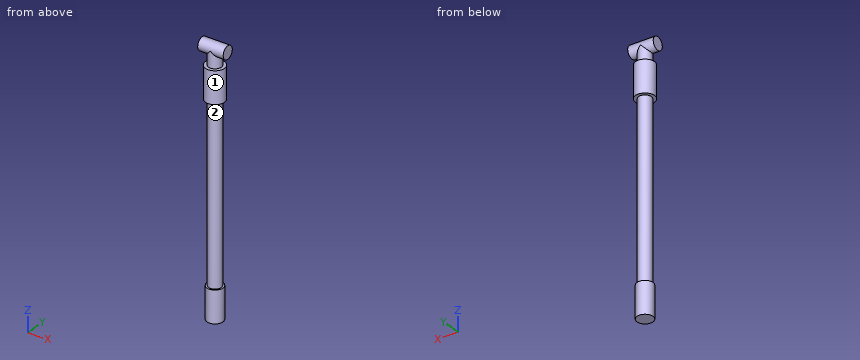
from build123d import *

# Parameters (mm, degrees)
SKETCH1_R                = 4
BOSS_EXTRUDE1_DEPTH      = 150
SKETCH2_R                = 5
BOSS_EXTRUDE2_DEPTH      = 20
SKETCH3_R                = 6
BOSS_EXTRUDE3_DEPTH      = 20
BOSS_EXTRUDE6_START      = 10
SKETCH4_R                = 4
BOSS_EXTRUDE6_DEPTH      = 10
BOSS_EXTRUDE7_DEPTH      = 8
BOSS_EXTRUDE7_DEPTH_BACK = 8
SKETCH6_R                = 4


with BuildPart() as part:
    # Sketch1 → Boss-Extrude1 (new body)
    with BuildSketch(Plane.XY):
        Circle(SKETCH1_R)
    extrude(amount=-BOSS_EXTRUDE1_DEPTH)

    # Sketch2 → Boss-Extrude2 (add)
    with BuildSketch(Plane(origin=(0, 0, -150), x_dir=(-1, 0, 0), z_dir=(0, 0, -1))):
        Circle(SKETCH2_R)
    extrude(amount=-BOSS_EXTRUDE2_DEPTH)

    # Sketch3 → Boss-Extrude3 (add)
    with BuildSketch(Plane.XY):
        Circle(SKETCH3_R)
    extrude(amount=-BOSS_EXTRUDE3_DEPTH)

    # Sketch4 → Boss-Extrude6 (add)
    with BuildSketch(Plane.XY.offset(BOSS_EXTRUDE6_START)):
        Circle(SKETCH4_R)
    extrude(amount=-BOSS_EXTRUDE6_DEPTH)

    # Sketch6 → Boss-Extrude7 (add, two sides: drawn at the far end of the back side and taken through both)
    with BuildSketch(Plane(origin=(0, 0, 0), x_dir=(0, 0, -1), z_dir=(1, 0, 0)).offset(-BOSS_EXTRUDE7_DEPTH_BACK)):
        with Locations((-10, 0)):
            Circle(SKETCH6_R)
    extrude(amount=BOSS_EXTRUDE7_DEPTH + BOSS_EXTRUDE7_DEPTH_BACK)


solid = part.part
Geometry: final body of the model. Coordinates: model frame, mm. Face numbers are marked on the shaded views. Round coordinates to 2 decimals unless told otherwise and drop trailing zeros. Loops run counter-clockwise (first coordinate to the right, second up) from the corner with the lowest first, then second, coordinate; pieces in that order, holes last. Notation, with made-up numbers: M 87.5,53 L 118.5,53 A16 cw 118.5,80 Z; hole C 47.5,36.25 d9. An arc over 180 degrees is marked long. One line per question, with ' | ' between items.
(1) Cut plane D-D on z = -100.5. Return the cut outline in (x, y).
Check result:
outline: C 0,0 d8
(2) Cut plane B-B on y = 0. Return the cut outline in (x, z).
Check result:
outline: M -8,6 L -4,6 L -4,0 L -6,0 L -6,-20 L -4,-20 L -4,-130 L -5,-130 L -5,-150 L 5,-150 L 5,-130 L 4,-130 L 4,-20 L 6,-20 L 6,0 L 4,0 L 4,6 L 8,6 L 8,14 L -8,14 Z
(3) Pull-direction query (Z, two-part tool) for the marked faces 1 and 2; classes: +Z half, -Z half, draft (parallel to the pull), parting line (faces both ways), or undercut.
Check result:
face 1: draft | face 2: undercut
(4) Cut plane A-A on x = 0. Return the cut outline in (y, z), plus the area to 3 significant figures.
Check result:
outline: M -6,-20 L -4,-20 L -4,-130 L -5,-130 L -5,-150 L 5,-150 L 5,-130 L 4,-130 L 4,-20 L 6,-20 L 6,0 L 4,0 L 4,10 A4 ccw -4,10 L -4,0 L -6,0 Z | area: 1,430 mm2
(5) Cut plane C-C on z = -132. Return the cut outline in (x, y), plus the area to 3 significant figures.
Check result:
outline: C 0,0 d10 | area: 78.5 mm2
(6) Material intervals for line 1 along X through (y, z) = (0.5, -49.5); line 2 along Z through (x, y) = (-3.75, 2.5), sorted ascending. Write a range as from..to.
Check result:
line 1: x = -3.97..3.97 | line 2: z = -150..-130, -20..0, 6.88..13.12
(7) Contact query for flat-ended pins moving along their axis: P1, Ø2, axis at x = 6, y = 2, coming from the +Z side; P2, Ø6, axis at x = -6, y = -2.5, coming from the -Z side; P3, Ø8, axis at x = 3.5, z = -48, coming from the -Y side; P4, Ø6, axis at x = 0.5, z = -50, coming from the +Y side. Output: stop coordinate, or through.
Check result:
P1: stops at z = 13.87 | P2: stops at z = -150 | P3: stops at y = -4 | P4: stops at y = 4
